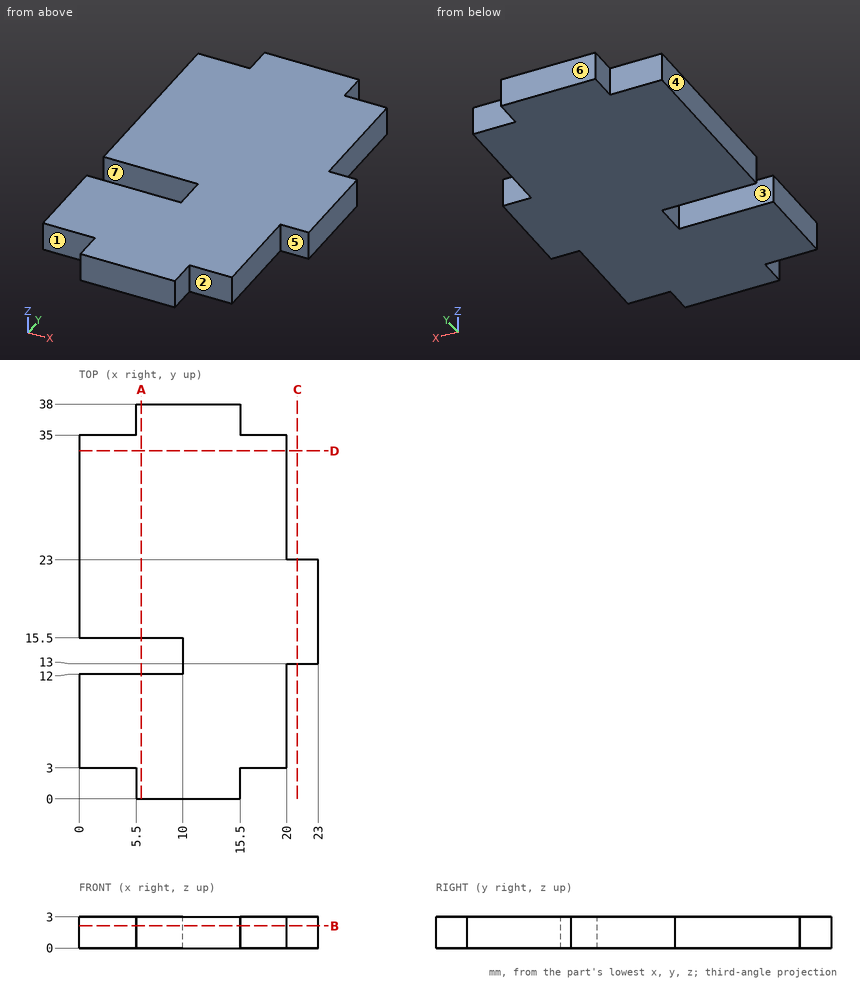
The drawing under review shows one solid part. Ordinate dimensions are in mm from its lowest x, y, z. A direction names the side the tool comes from. Round coordinates to 2 decimals unless told otherwise and drop trailing zeros. Order: outer loops, then holes, each group sorted by start corner. A loop starts at its lowest first (then second) coordinate and runs counter-clockwise, first axis right, second up. Notation, with made-up numbers: (-16, 80.25) - (23, 80.25) arc R17 cw to (23, 88.25) - close; hole circle Ø5 at (41.5, 3). An arc over 180 degrees is marked (long way). Return JSON: item names as keys, results as strings.
Q1. The part is to be moulded in two halves that separate along Y. For the marked faces 4, 5, 6 and 7, say which applies: pulls with the +Y half, pulls with the -Y half, needs draft (parallel to the pull), parting line crosses it, or undercut.
Computed values:
{"face 4": "needs draft", "face 5": "pulls with the -Y half", "face 6": "pulls with the +Y half", "face 7": "undercut"}
Q2. Consider section B-B on z = 2.15. Write out the cut boundary in (x, y).
Computed values:
{"outline": "(0, 3) - (5.5, 3) - (5.5, 0) - (15.5, 0) - (15.5, 3) - (20, 3) - (20, 13) - (23, 13) - (23, 23) - (20, 23) - (20, 35) - (15.5, 35) - (15.5, 38) - (5.5, 38) - (5.5, 35) - (0, 35) - (0, 15.5) - (10, 15.5) - (10, 12) - (0, 12) - close"}
Q3. Consider section C-C on x = 21. Write out the cut boundary in (y, z).
Computed values:
{"outline": "(13, 0) - (23, 0) - (23, 3) - (13, 3) - close"}
Q4. Wall thickness on L1, parallel to Y at x = 2.5, z = 1; L2, parallel to Y at x = 8.75, z = 0.55; L3, parallel to Y at x = 21, z = 0.9: over which ranges is each line inside the solid? List them lowest first. Write a range as [from, to].
Computed values:
{"L1": "y = [3, 12], [15.5, 35]", "L2": "y = [0, 12], [15.5, 38]", "L3": "y = [13, 23]"}
Q5. Consider section D-D on y = 33.5. Write out the cut boundary in (x, z), plus the area to 3 significant figures.
Computed values:
{"outline": "(0, 0) - (20, 0) - (20, 3) - (0, 3) - close", "area": "60.0 mm2"}
Q6. Machinability: for the marked faces 1, 2 and 3, which of the approach directions +Z, -Z, +X, -X, +Y, -Y give a long, thin tool a straight path to every point of the face, cutting with its end or side? Answer none if there is none.
Computed values:
{"face 1": "+Z, -Z, -X, -Y", "face 2": "+Z, -Z, +X, -Y", "face 3": "+Z, -Z, -X"}
Q7. For pin 1 Ø0.9 at (x, z) = (5, 1) entering from -Y; pin 2 Ø1.5 at (x, z) = (4.5, 2) entering from +Y; pin 3 Ø1.5 at (y, z) = (31, 1.5) entering from +X, all flat-tipped, find the tip position at first contact; note any pin that passes through.
Computed values:
{"pin 1": "stops at y = 3", "pin 2": "stops at y = 35", "pin 3": "stops at x = 20"}
Q8. Consider section A-A on x = 6. Write out the cut boundary in (y, z).
Computed values:
{"outline": "(0, 0) - (12, 0) - (12, 3) - (0, 3) - close; (15.5, 0) - (38, 0) - (38, 3) - (15.5, 3) - close"}
